Geometry check sheet. Reference: the model listing, model coordinates, mm. Face numbers are marked on the shaded views. A direction names the side the tool comes from. Coordinates: 2 decimals unless noted, no trailing zeros. Write each loop counter-clockwise with the first axis right and the second up, starting at its lowest first coordinate (ties: lowest second). Pieces come first, ordered by that corner, then holes. Notation, with made-up numbers: (-9, 6.25) -> (2, 6.25) arc R9 cw to (2, 21.25) -> close; hole circle Ø8 at (23.5, 5.25). An arc over 180 degrees is marked (long way). Answer in a Markdown table with one row per item. Add a question column.
Q1. Section check C-C, the plane y = 1. Record the boundary of the cut face in (x, z).
Q2. Tool access check on the marked faces 5, 6 and 7. Record the directions out of +Z, -Z, +X, -X, +Y, -Y that give a thin tool (end or side, any length) a straight path to the whole face; none if there is none.
Q3. Thickness scan on line 1 (X direction, y = -9, z = 23); line 2 (Z direction, x = 3, y = -8.5); line 3 (Y direction, x = 10, z = 14). Record the ranges inside material, lowest first.
Q4. Section check A-A, the plane z = 18.5. Record the boundary of the cut face in (x, y), and give its area (3 significant figures).
Q5. Section check D-D, the plane z = 27.5. Record the boundary of the cut face in (x, y).
Q6. Gauge pin test, flat ends, axial feed: P1, Ø9, axis at x = 9, z = 15, coming from the +Y side; P2, Ø12, axis at y = 5.5, z = 28, coming from the +X side; P3, Ø4, axis at x = 13, y = -30.5, coming from the +Z side; P4, Ø8, axis at y = -5, z = 12, coming from the -X side. Record the tip position at first contact, or that the pin passes through.
Q7. Release check for a two-part mould opening along X. For the marked faces 1, 2, 3 and 4 record: pulls with the +X half, pulls with the -X half, needs draft (parallel to the pull), parting line crosses it, or undercut.
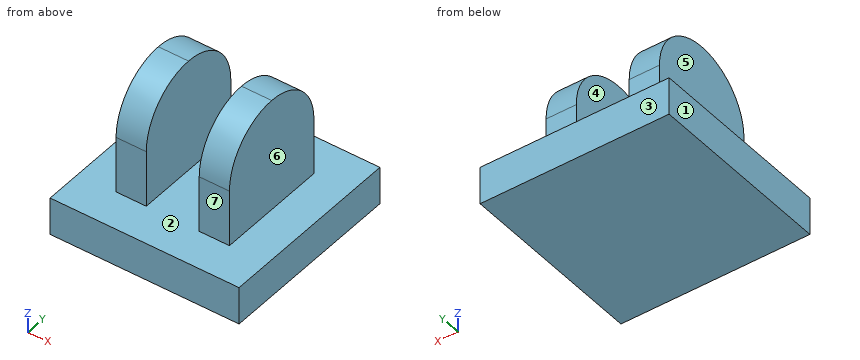
```python
from build123d import *

# Parameters (mm, degrees)
F0_W     = 50
F0_H     = 50
F3_DEPTH = 10
F2_W     = 8
F2_H     = 30
F4_DEPTH = 40
F1_W     = 8
F1_H     = 30
F5_DEPTH = 40
F6_R     = 14.99999
F7_R     = 14.99999


# Not quite as in the source:
# - a fillet or chamfer is up to 0.001 mm smaller than in the source, because OpenCascade refuses the exact size


with BuildPart() as f3:
    # F0 (on Top) → F3 (new body)
    with BuildSketch(Plane.XY):
        with Locations((-0.7709864527, -12.4589413404)):
            Rectangle(F0_W, F0_H)
    extrude(amount=F3_DEPTH)

    # F2 (on face) → F4 (join)
    with BuildSketch(Plane.XY):
        with Locations((10.2290135473, -12.4589413404)):
            Rectangle(F2_W, F2_H)
    extrude(amount=F4_DEPTH)

    # F1 (on face) → F5 (join)
    with BuildSketch(Plane.XY):
        with Locations((-11.7709864527, -12.4589413404)):
            Rectangle(F1_W, F1_H)
    extrude(amount=F5_DEPTH)

    # F6 (radius 15 in the source; OpenCascade refuses exactly that, so slightly less here)
    f6_edges = [f3.edges().sort_by_distance(p)[0] for p in [
        (-11.770986, -27.458941, 40),
        (-11.770986, 2.541059, 40),
    ]]
    fillet(f6_edges, radius=F6_R)

    # F7 (radius 15 in the source; OpenCascade refuses exactly that, so slightly less here)
    f7_edges = [f3.edges().sort_by_distance(p)[0] for p in [
        (10.229014, 2.541059, 40),
        (10.229014, -27.458941, 40),
    ]]
    fillet(f7_edges, radius=F7_R)


solid = f3.part
```
Calculated:
| question | item | result |
|---|---|---|
| 1 | outline | (-25.77, 0) -> (24.23, 0) -> (24.23, 10) -> (14.23, 10) -> (14.23, 31.62) -> (6.23, 31.62) -> (6.23, 10) -> (-7.77, 10) -> (-7.77, 31.62) -> (-15.77, 31.62) -> (-15.77, 10) -> (-25.77, 10) -> close |
| 2 | face 5 | +Z, -X, +Y, -Y |
| 2 | face 6 | +Z, +X, +Y, -Y |
| 2 | face 7 | +Z, +X, -X, -Y |
| 3 | line 1 | x = -15.77 to -7.77, 6.23 to 14.23 |
| 3 | line 2 | z = 0 to 10 |
| 3 | line 3 | y = -27.46 to 2.54 |
| 4 | outline | (-15.77, -27.46) -> (-7.77, -27.46) -> (-7.77, 2.54) -> (-15.77, 2.54) -> close; (6.23, -27.46) -> (14.23, -27.46) -> (14.23, 2.54) -> (6.23, 2.54) -> close |
| 4 | area | 480 mm² |
| 5 | outline | (-15.77, -27.25) -> (-7.77, -27.25) -> (-7.77, 2.33) -> (-15.77, 2.33) -> close; (6.23, -27.25) -> (14.23, -27.25) -> (14.23, 2.33) -> (6.23, 2.33) -> close |
| 6 | P1 | stops at y = 2.54 |
| 6 | P2 | stops at x = 14.23 |
| 6 | P3 | stops at z = 10 |
| 6 | P4 | stops at x = -25.77 |
| 7 | face 1 | pulls with the -X half |
| 7 | face 2 | undercut |
| 7 | face 3 | needs draft |
| 7 | face 4 | undercut |
